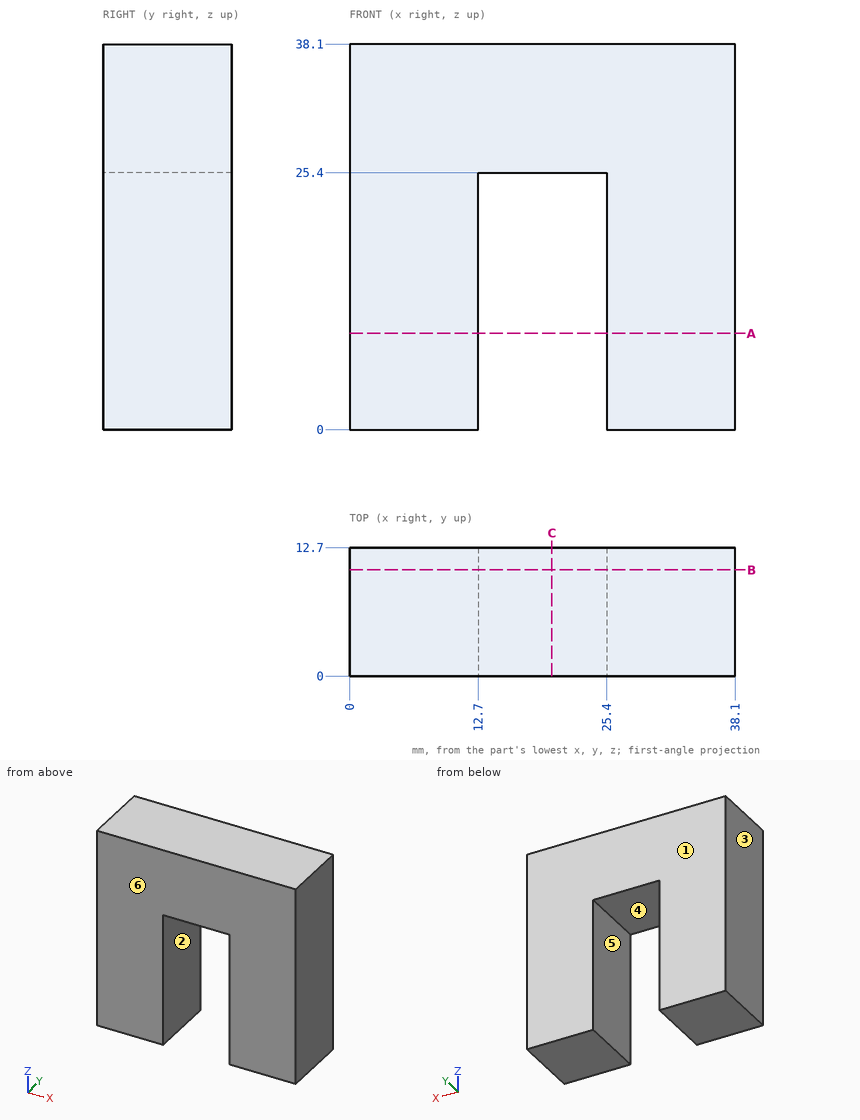
Answer from the drawing. Dimensions are ordinates in mm from the lowest x, y and z of the part. A direction names the side the tool comes from. Give positions to 0.01 mm unless a question says otherwise; leave off trailing zeros. Order: outer loops, then holes, each group sorted by start corner. A loop starts at its lowest first (then second) coordinate and runs counter-clockwise, first axis right, second up.
(1) Find section B-B (y = 10.5). Give the vertices of the cut face in (x, z).
(2) Straight lines are drawn through the part: L1, parallel to X at y = 6.75, z = 12; L2, parallel to Z at x = 15.5, y = 11. For each, find the intervals that lie inside material, in ascending order.
(3) Find section C-C (x = 20). Give the vertices of the cut face in (y, z), plus the area to 3 significant figures.
(4) For a pull along X with two mould halves and no side action, classify the marked faces 1, 2, 3 and 4 as released by +X, released by -X, zero draft, split by the parting line, or undercut.
(5) For the marked faces 5 and 6, determine the directions among +Z, -Z, +X, -X, +Y, -Y from which every point of the face is accessible in a straight line to the end or side of a thin tool.
(6) Given pin 1 (6.5 mm diameter, centred on x = 21.5, y = 3.5, fed in from -Z), flat-ended and moving along its own axis, determine where the tip first touches the part or whether it passes through.
(7) Find section A-A (z = 9.5). Give the vertices of the cut face in (x, y), plus the area to 3 significant figures.
Result sheet:
1. outline: (0, 0) - (12.7, 0) - (12.7, 25.4) - (25.4, 25.4) - (25.4, 0) - (38.1, 0) - (38.1, 38.1) - (0, 38.1) - close
2. L1: x = 0 to 12.7, 25.4 to 38.1
2. L2: z = 25.4 to 38.1
3. outline: (0, 25.4) - (12.7, 25.4) - (12.7, 38.1) - (0, 38.1) - close
3. area: 161 mm2
4. face 1: zero draft
4. face 2: undercut
4. face 3: released by -X
4. face 4: undercut
5. face 5: -Z, +Y, -Y
5. face 6: +Z, -Z, +X, -X, -Y
6. pin 1: stops at z = 25.4
7. outline: (0, 0) - (12.7, 0) - (12.7, 12.7) - (0, 12.7) - close; (25.4, 0) - (38.1, 0) - (38.1, 12.7) - (25.4, 12.7) - close
7. area: 323 mm2
